```python
from build123d import *

# Parameters (mm, degrees)
SKETCH1_R           = 6.25
BOSS_EXTRUDE1_DEPTH = 14
SKETCH2_R           = 2.6
CUT_EXTRUDE1_DEPTH  = 14
CUT_EXTRUDE2_DEPTH  = 7
SKETCH4_R           = 4.5
CUT_EXTRUDE3_DEPTH  = 4


with BuildPart() as part:
    # Sketch1 → Boss-Extrude1 (new body)
    with BuildSketch(Plane(origin=(0, 0, 0), x_dir=(1, 0, 0), z_dir=(0, 1, 0))):
        Circle(SKETCH1_R)
    extrude(amount=BOSS_EXTRUDE1_DEPTH)

    # Sketch2 → Cut-Extrude1 (cut)
    with BuildSketch(Plane(origin=(0, 14, 0), x_dir=(1, 0, 0), z_dir=(0, 1, 0))):
        Circle(SKETCH2_R)
    extrude(amount=-CUT_EXTRUDE1_DEPTH, mode=Mode.SUBTRACT)

    # Sketch3 → Cut-Extrude2 (cut, symmetric)
    with BuildSketch(Plane(origin=(0, 0, 0), x_dir=(0, 0, -1), z_dir=(1, 0, 0))):
        Polygon((2.25, 14), (6.25, 10), (6.25, 14), align=None)
    extrude(amount=CUT_EXTRUDE2_DEPTH, both=True, mode=Mode.SUBTRACT)

    # Sketch4 → Cut-Extrude3 (cut)
    with BuildSketch(Plane.XZ):
        Circle(SKETCH4_R)
    extrude(amount=-CUT_EXTRUDE3_DEPTH, mode=Mode.SUBTRACT)


solid = part.part
```
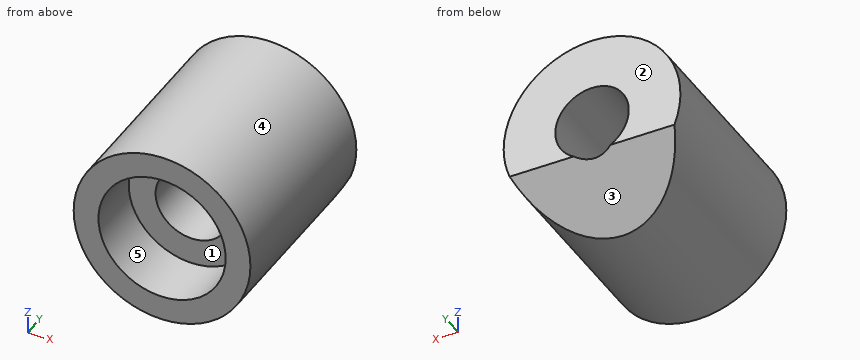
Design review of the part built by this model. Coordinates are the model's own, in mm. Face numbers are marked on the shaded views. A direction names the side the tool comes from. Give positions to 0.01 mm unless a question says otherwise; leave off trailing zeros. Order: outer loops, then holes, each group sorted by start corner. A loop starts at its lowest first (then second) coordinate and runs counter-clockwise, first axis right, second up. Notation, with made-up numbers: (28, 47) - (48, 47) arc R24 ccw to (48, 58) - close; hole circle Ø4 at (-4, 42). An arc over 180 degrees is marked (long way). Use a Markdown table: item, result. Add a question column.
(1) Add section B-B on z = 0. Give the boundary of the cut face in (x, y).
(2) Add section D-D on x = -3. Give the boundary of the cut face in (y, z).
(3) Mouldability with a two-part tool opening along X and no side actions: class the marked faces 3, 4 and 5 as +X half, -X half, draft (parallel to the pull), parting line (faces both ways), or undercut.
(4) Machinability: for the marked faces 1 and 2, which of the approach directions +Z, -Z, +X, -X, +Y, -Y give a long, thin tool a straight path to every point of the face, cutting with its end or side? Answer none if there is none.
(5) Clearance check with flat-ended pins moving along their axes: P1, Ø1, axis at x = -3, y = 2.5, coming from the -Z side; P2, Ø4.5, axis at x = 0.5, z = 1.5, coming from the -Y side; P3, Ø3, axis at x = 0, z = 0, coming from the +Y side; P4, Ø1.5, axis at x = 3.5, y = 7.5, coming from the +Z side. State where each tip first meets the part, or that it passes through.
(6) Add section A-A on x = 0. Give the boundary of the cut face in (y, z), then the cut area to 3 significant figures.
(7) Wall thickness on probe 1 along X at (y, z) = (6.75, 0); probe 2 along Z at (x, y) = (0, 2.65): over which ranges is each line inside the solid? List them lowest first. Write a range as [from, to].
(8) Add section C-C on y = 7. Give the boundary of the cut face in (x, z).
Report:
| question | item | result |
|---|---|---|
| 1 | outline | (-6.25, 0) - (-4.5, 0) - (-4.5, 4) - (-2.6, 4) - (-2.6, 14) - (-6.25, 14) - close; (2.6, 4) - (4.5, 4) - (4.5, 0) - (6.25, 0) - (6.25, 14) - (2.6, 14) - close |
| 2 | outline | (0, -5.48) - (10.77, -5.48) - (14, -2.25) - (14, 5.48) - (0, 5.48) - (0, 3.35) - (4, 3.35) - (4, -3.35) - (0, -3.35) - close |
| 3 | face 3 | draft |
| 3 | face 4 | parting line |
| 3 | face 5 | undercut |
| 4 | face 1 | -Y |
| 4 | face 2 | +Z, -Z, +X, -X, +Y |
| 5 | P1 | stops at z = -5.73 |
| 5 | P2 | stops at y = 4 |
| 5 | P3 | passes through |
| 5 | P4 | stops at z = 5.61 |
| 6 | outline | (0, -6.25) - (10, -6.25) - (13.65, -2.6) - (4, -2.6) - (4, -4.5) - (0, -4.5) - close; (0, 4.5) - (4, 4.5) - (4, 2.6) - (14, 2.6) - (14, 6.25) - (0, 6.25) - close |
| 6 | area | 79.1 mm² |
| 7 | probe 1 | x = [-6.25, -2.6], [2.6, 6.25] |
| 7 | probe 2 | z = [-6.25, -4.5], [4.5, 6.25] |
| 8 | outline | circle Ø12.5 at (0, 0); hole circle Ø5.2 at (0, 0) |
